Read the model definition and answer for the solid it produces. Units are mm, in the model's axes. A direction names the side the tool comes from. Coordinates: 2 decimals unless noted, no trailing zeros. Write each loop counter-clockwise with the first axis right and the second up, starting at its lowest first coordinate (ties: lowest second). Pieces come first, ordered by that corner, then holes. Notation, with made-up numbers: (27.5, -34) -> (83.5, -34) arc R23 ccw to (83.5, 4) -> close; hole circle Ø9 at (72, 34.5). An arc over 180 degrees is marked (long way). Return JSON: item names as keys, results as strings.
from build123d import *

# Parameters (mm, degrees)
EXTRUDE_1_DEPTH     = 70
SKETCH_2_R          = 2.25
CUT_EXTRUDE_1_DEPTH = 2
SKETCH_3_R          = 2.25
CUT_EXTRUDE_2_DEPTH = 2


with BuildPart() as part:
    # Эскиз1 → Бобышка-Вытянуть1 (new body)
    with BuildSketch(Plane.XY):
        Polygon((0, 0), (0, 20), (1, 20), (1, 1), (20, 1), (20, 0), align=None)
    extrude(amount=EXTRUDE_1_DEPTH)

    # Эскиз2 → Вырез-Вытянуть1 (cut, through all)
    with BuildSketch(Plane(origin=(0, 1, 0), x_dir=(1, 0, 0), z_dir=(0, 1, 0))):
        with Locations((10.5, -10)):
            Circle(SKETCH_2_R)
        with Locations((10.5, -60)):
            Circle(SKETCH_2_R)
    extrude(amount=-CUT_EXTRUDE_1_DEPTH, mode=Mode.SUBTRACT)

    # Эскиз3 → Вырез-Вытянуть2 (cut, through all)
    with BuildSketch(Plane(origin=(1, 0, 0), x_dir=(0, 0, -1), z_dir=(1, 0, 0))):
        with Locations((-10, 15)):
            Circle(SKETCH_3_R)
        with Locations((-60, 15)):
            Circle(SKETCH_3_R)
    extrude(amount=-CUT_EXTRUDE_2_DEPTH, mode=Mode.SUBTRACT)


solid = part.part
1. The part is cut by section A-A (z = 60). Determine the outline of the cut face in (x, y).
Taken from the geometry:
{"outline": "(0, 0) -> (8.25, 0) -> (8.25, 1) -> (1, 1) -> (1, 12.75) -> (0, 12.75) -> close; (0, 17.25) -> (1, 17.25) -> (1, 20) -> (0, 20) -> close; (12.75, 0) -> (20, 0) -> (20, 1) -> (12.75, 1) -> close"}
2. For a pull along Z with two mould halves and no side action, classify faces 3 (the face through (0.507, 15.099, 62.248)), 4 (the face through (1, 11, 35)), 5 (the face through (5.6, 0.4, 70)), 6 (the face through (0.507, 12.804, 10.488)) as +Z half, -Z half, draft (parallel to the pull), parting line (faces both ways), or undercut.
Taken from the geometry:
{"face 3": "undercut", "face 4": "draft", "face 5": "+Z half", "face 6": "undercut"}
3. A tool of negligible diameter and unlimited length cuts with its end or side. For faces 1 (the face through (5.6, 0.4, 0)), 2 (the face through (10, 1, 35)), from which of +Z, -Z, +X, -X, +Y, -Y can it reach the whole face along a straight path? Write none if from no direction.
Taken from the geometry:
{"face 1": "-Z, +X, -X, +Y, -Y", "face 2": "+Z, -Z, +X, +Y"}
4. The part is cut by section C-C (z = 47). Determine the outline of the cut face in (x, y).
Taken from the geometry:
{"outline": "(0, 0) -> (20, 0) -> (20, 1) -> (1, 1) -> (1, 20) -> (0, 20) -> close"}
5. Consider L1, parallel to Z at x = 10.5, y = 0.8; L2, parallel to X at y = 0.8, z = 60; L3, parallel to Y at x = 0.55, z = 60. Determine where each line is inside the solid, lowest interval first.
Taken from the geometry:
{"L1": "z = 0 to 7.75, 12.25 to 57.75, 62.25 to 70", "L2": "x = 0 to 8.25, 12.75 to 20", "L3": "y = 0 to 12.75, 17.25 to 20"}
6. The part is cut by section D-D (y = 6.25). Determine the outline of the cut face in (x, z), then the cut area to 3 significant figures.
Taken from the geometry:
{"outline": "(0, 0) -> (1, 0) -> (1, 70) -> (0, 70) -> close", "area": "70.0 mm2"}
7. Flat-ended cylindrical pins translate along their axes: pin 1 Ø8 at (y, z) = (15.5, 37.5) entering from +X; pin 2 Ø3.5 at (y, z) = (15, 60) entering from +X; pin 3 Ø9.5 at (x, z) = (12.5, 38) entering from +Y. Find the tip coordinate at first contact, or state that the pin passes through.
Taken from the geometry:
{"pin 1": "stops at x = 1", "pin 2": "passes through", "pin 3": "stops at y = 1"}
8. The part is cut by section B-B (x = 10.5). Determine the outline of the cut face in (y, z).
Taken from the geometry:
{"outline": "(0, 0) -> (1, 0) -> (1, 7.75) -> (0, 7.75) -> close; (0, 12.25) -> (1, 12.25) -> (1, 57.75) -> (0, 57.75) -> close; (0, 62.25) -> (1, 62.25) -> (1, 70) -> (0, 70) -> close"}
